Autodesk Inventor part; units mm, degrees
ref_plane "YZ Plane" through (0, 0, 0) normal (1, 0, 0) x (0, 1, 0)
ref_plane "XZ Plane" through (0, 0, 0) normal (0, 1, 0) x (-1, 0, 0)
ref_plane "XY Plane" through (0, 0, 0) normal (0, 0, 1) x (1, 0, 0)
sketch "Esboço1" plane through (0, 0, 0) normal (0, 1, 0) x (-1, 0, 0)
  line L0 (0, 0) -> (200, 0)
  line L1 (200, 0) -> (200, -100)
  line L2 (200, -100) -> (300, -100)
  line L3 (300, -100) -> (300, -200)
  line L4 (300, -200) -> (0, -200)
  line L5 (0, -200) -> (0, 0)
  dimension "d0" = 200
  dimension "d1" = 300
  dimension "d3" = 200
  dimension "d4" = 100
extrude "Extrusão1" add sketch "Esboço1" along normal blind 50
sketch "Esboço2" plane through (0, 50, 0) normal (0, 1, 0) x (1, 0, 0)
  line L0 (0, 0) -> (0, 200)
  line L1 (0, 200) -> (-300, 200)
  point P0 (-100, 100)
  dimension "d7" = 100
  dimension "d15" = 100
hole "Furo1" at (-100, 50, -100) direction (0, -1, 0) diameter 100 end through all counterbore diameter 150 counterbore depth 25
fillet "Arredondamento1" radius 50 2 edges at (0, 25, 0) (0, 25, -200)
fillet "Arredondamento2" radius 30 1 edges at (-200, 25, -100)
chamfer "Chanfro1" distance 25 angle 45 1 edges at (-300, 25, -100) measured on face at (-276.6667, 16.6667, -100)
equation "\"d16\" = 0.25 * d3"
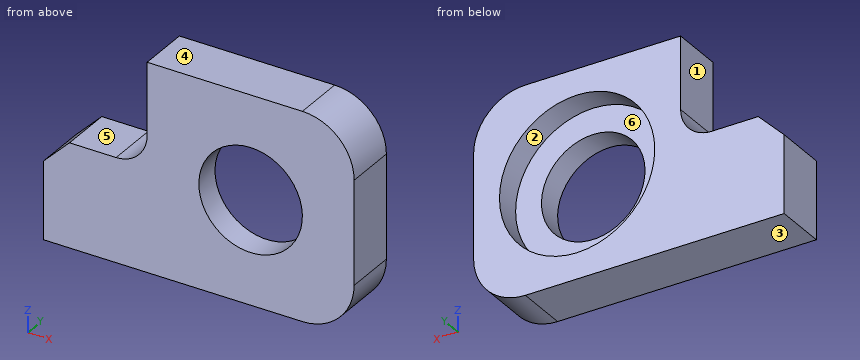
Could you check a few things on this model? Use its own coordinates, in mm. Face numbers are marked on the shaded views. A direction names the side the tool comes from. Round coordinates to 2 decimals unless told otherwise and drop trailing zeros. Order: outer loops, then holes, each group sorted by start corner. A loop starts at its lowest first (then second) coordinate and runs counter-clockwise, first axis right, second up.
(1) Please list where these lines run through material, in increasing order: line 1 along Z through (x, y) = (-100, 13); line 2 along Z through (x, y) = (-99, 25.5); line 3 along Z through (x, y) = (-268.5, 17).
Response values:
line 1: z = -200 to -150, -50 to 0
line 2: z = -200 to -174.99, -25.01 to 0
line 3: z = -200 to -100
(2) I'm going to push flat-ended pins straight in: pin 1 (25 mm diameter, centred on y = 21.5, z = -20.5, fed in from -X); pin 2 (2 mm diameter, centred on x = -156, z = -161, fed in from -Y); pin 3 (8 mm diameter, centred on x = -262, y = 14, fed in from +Z). Where does each tip first touch, or does it pass through?
Response values:
pin 1: stops at x = -200
pin 2: stops at y = 0
pin 3: stops at z = -100
(3) Imagine slicing it at C-C (z = -110). Write out the boundary of the cut face in (x, y), plus the area to 3 significant figures.
Response values:
outline: (-285, 0) - (-148.99, 0) - (-148.99, 25) - (-174.33, 25) - (-174.33, 50) - (-285, 50) - close; (-51.01, 0) - (0, 0) - (0, 50) - (-25.67, 50) - (-25.67, 25) - (-51.01, 25) - close
area: 8,080 mm2
(4) If we mould it in two halves opening along Z, with no side actions, what happens to the marked faces 1, 2 and 3? For each: released by +Z, released by -Z, zero draft, split by the parting line, or undercut.
Response values:
face 1: zero draft
face 2: undercut
face 3: released by -Z
(5) Imagine slicing it at A-A (x = -100). Write out the boundary of the cut face in (y, z).
Response values:
outline: (0, -200) - (50, -200) - (50, -175) - (25, -175) - (25, -150) - (0, -150) - close; (0, -50) - (25, -50) - (25, -25) - (50, -25) - (50, 0) - (0, 0) - close
(6) Imagine slicing it at B-B (y = 7). Write out the boundary of the cut face in (x, z), plus the area to 3 significant figures.
Response values:
outline: (-300, -200) - (-50, -200) arc R50 ccw to (0, -150) - (0, -50) arc R50 ccw to (-50, 0) - (-200, 0) - (-200, -70) arc R30 cw to (-230, -100) - (-275, -100) - (-300, -125) - close; hole circle Ø100 at (-100, -100)
area: 41,000 mm2
(7) Which directions (+Z, -Z, +X, -X, +Y, -Y) give clear straight access to the entire face, cutting with the end or side of a thin tool? Please do the marked faces 4, 5 and 6.
Response values:
face 4: +Z, +X, -X, +Y, -Y
face 5: +Z, -X, +Y, -Y
face 6: +Y
